```python
from build123d import *

# Parameters (mm, degrees)
REVOLVE1_ANGLE = 359.999999589


with BuildPart() as part:
    # Sketch1 → Revolve1 (revolve)
    with BuildSketch(Plane.XY):
        Polygon((0, 0), (250, 200), (550, 380), (850, 500), (900, 540), (920, 540), (920, 460), (850, 460), (550, 350), (250, 170), (50, 0), align=None)
    revolve(axis=Axis((0, 0, 0), (1, 0, 0)), revolution_arc=REVOLVE1_ANGLE)


solid = part.part
```
Input: part model. Units: mm. Frame: model coordinates. A direction names the side the tool comes from. Give positions to 0.01 mm unless a question says otherwise; leave off trailing zeros. Write each question's results on one line, items separated by ' | '. Start each with the question number.
Item 1: Line query: line 1 (Z direction, x = 896, y = 0); line 2 (Y direction, x = 332.5, z = -14); line 3 (Z direction, x = 891.5, y = 0). Output: solid intervals per line, ascending.
Item 2: Contact query for flat-ended pins moving along their axis: P1, Ø6, axis at x = 211, y = -128.5, coming from the -Z side; P2, Ø3, axis at y = 311.5, z = 309.5, coming from the -X side; P3, Ø6, axis at y = 33, z = 75.5, coming from the +X side. Output: stop coordinate, or through.
Item 3: Mould query, pull axis Y, two halves, no side actions, for faces 1 (the conical face through (104.16, -45.99, 2.02)), 2 (the conical face through (568.767, -387.132, 17.038)), 3 (the conical face through (564.57, -355, 15.62)), 4 (the flat face through (920, 397, 243)). Classes: pulls with the +Y half, pulls with the -Y half, needs draft (parallel to the pull), parting line crosses it, or undercut.
Item 4: Set-up query: faces 5 (the cylindrical face through (884.51, -459.555, 20.225)), 6 (the conical face through (71.194, -56.9, 2.504)). Return all of +Z, -Z, +X, -X, +Y, -Y with unobstructed straight access to the full face (end or side cutting, diameter ignored); none if empty.
Established:
1) line 1: -536.8 to -460, 460 to 536.8 | line 2: -249.11 to -219.05, 219.05 to 249.11 | line 3: -533.2 to -460, 460 to 533.2
2) P1: z = -114.45 | P2: x = 694.04 | P3: x = 150.47
3) face 1: undercut | face 2: parting line crosses it | face 3: undercut | face 4: needs draft
4) face 5: +X | face 6: -X
